Design review of the part built by this model. Coordinates are the model's own, in mm. Coordinates: 2 decimals unless noted, no trailing zeros. Loops run counter-clockwise (first coordinate to the right, second up) from the corner with the lowest first, then second, coordinate; pieces in that order, holes last. Notation, with made-up numbers: (71.5, 43) -> (101.5, 43) arc R27 cw to (101.5, 71) -> close; hole circle Ø2 at (30, -2.5). An arc over 180 degrees is marked (long way). Use a Markdown table: item, result. Add a question column.
Q1. For probe 1 along X at (y, z) = (-0.75, -127); probe 2 along Y at (x, z) = (278.5, -21.5); probe 3 along X at (y, z) = (-2, -63) (3 decimals), list the stretches that pass through material, from the lowest coordinate up.
Q2. Take a section at A-A on x = 1294. Write out the cut boundary in (y, z) (3 decimals), plus the area to 3 significant figures.
Q3. Clearance check with flat-ended pins moving along their axes: pin 1 Ø9 at (x, z) = (1057.275, -22.225) entering from -Y; pin 2 Ø2 at (y, z) = (-2, -117) entering from +X; pin 3 Ø1.3 at (x, y) = (677, 34) entering from -Z; pin 4 Ø8 at (x, z) = (930.275, -127) entering from +Y. State where each tip first meets the part, or that it passes through.
from build123d import *

# Parameters (mm, degrees)
BASE_FLANGE1_DEPTH               = 2.65684
EDGE_FLANGE3_STRIP_W             = 16.97736
EDGE_FLANGE3_STRIP_H             = 2.65684
EDGE_FLANGE3_STRIP_CUT_DEPTH     = 1409.7
EDGE_FLANGE3_DEPTH               = 1409.7
EDGE_FLANGE4_STRIP_W             = 16.97736
EDGE_FLANGE4_STRIP_H             = 2.65684
EDGE_FLANGE4_STRIP_CUT_DEPTH     = 1409.7
EDGE_FLANGE4_DEPTH               = 1409.7
F_10_0_1935_DIAMETER_HOLE1_D     = 4.9149
F_17_64_0_26563_DIAMETER_HOLE1_D = 6.747002
FILLET1_R                        = 3.175


# Sheet-metal steps are written as plain solids
with BuildPart() as part:
    # Sketch1 → Base-Flange1 (new body)
    with BuildSketch(Plane(origin=(0, 0, 0), x_dir=(1, 0, 0), z_dir=(0, 1, 0))):
        Polygon((0, 0), (1409.7, 0), (1409.7, 38.1), (996.95, 38.1), (958.85, 88.9), (958.85, 139.7), (920.75, 139.7), (920.75, 88.9), (882.65, 38.1), (527.05, 38.1), (488.95, 88.9), (488.95, 139.7), (450.85, 139.7), (450.85, 88.9), (412.75, 38.1), (0, 38.1), align=None)
    extrude(amount=-BASE_FLANGE1_DEPTH)

    # Edge-Flange3 strip (across the edge) → Edge-Flange3 strip cut (cut)
    with BuildSketch(Plane(origin=(0, 0, 0), x_dir=(0, 0, -1), z_dir=(1, 0, 0))):
        with Locations((-2.65684, -1.32842)):
            Rectangle(EDGE_FLANGE3_STRIP_W, EDGE_FLANGE3_STRIP_H)
    extrude(amount=EDGE_FLANGE3_STRIP_CUT_DEPTH, mode=Mode.SUBTRACT)

    # Edge-Flange3 section (across the edge) → Edge-Flange3 (add)
    with BuildSketch(Plane(origin=(0, 0, 0), x_dir=(0, 0, -1), z_dir=(1, 0, 0))):
        with BuildLine():
            Line((0, 3.175), (0, 35.44316))
            Line((0, 35.44316), (2.65684, 35.44316))
            Line((2.65684, 35.44316), (2.65684, 3.175))
            ThreePointArc((2.65684, 3.175), (3.58677597, 0.92993597), (5.83184, 0))
            Line((5.83184, 0), (5.83184, -2.65684))
            ThreePointArc((5.83184, -2.65684), (1.708106389, -0.948733611), (0, 3.175))
        make_face()
    extrude(amount=EDGE_FLANGE3_DEPTH)

    # Edge-Flange4 strip (across the edge) → Edge-Flange4 strip cut (cut)
    with BuildSketch(Plane(origin=(0, 35.44316, -2.65684), x_dir=(0, -1, 0), z_dir=(1, 0, 0))):
        with Locations((-2.65684, -1.32842)):
            Rectangle(EDGE_FLANGE4_STRIP_W, EDGE_FLANGE4_STRIP_H)
    extrude(amount=EDGE_FLANGE4_STRIP_CUT_DEPTH, mode=Mode.SUBTRACT)

    # Edge-Flange4 section (across the edge) → Edge-Flange4 (add)
    with BuildSketch(Plane(origin=(0, 35.44316, -2.65684), x_dir=(0, -1, 0), z_dir=(1, 0, 0))):
        with BuildLine():
            Line((0, 3.175), (0, 35.44316))
            Line((0, 35.44316), (2.65684, 35.44316))
            Line((2.65684, 35.44316), (2.65684, 3.175))
            ThreePointArc((2.65684, 3.175), (3.58677597, 0.92993597), (5.83184, 0))
            Line((5.83184, 0), (5.83184, -2.65684))
            ThreePointArc((5.83184, -2.65684), (1.708106389, -0.948733611), (0, 3.175))
        make_face()
    extrude(amount=EDGE_FLANGE4_DEPTH)

    # #10 (0.1935) Diameter Hole1 (through all)
    with Locations(Plane(origin=(0, -2.65684, 0), x_dir=(-1, 0, 0), z_dir=(0, -1, 0))):
        with Locations((-460.375, 127), (-479.425, 127), (-460.375, 63.5), (-479.425, 63.5), (-460.375, 95.25), (-479.425, 95.25), (-930.275, 63.5), (-949.325, 63.5), (-930.275, 95.25), (-949.325, 95.25), (-949.325, 127), (-930.275, 127)):
            Hole(F_10_0_1935_DIAMETER_HOLE1_D / 2)

    # 17/64 (0.26563) Diameter Hole1 (through all)
    with Locations(Plane(origin=(0, 35.44316, 0), x_dir=(1, 0, 0), z_dir=(0, 1, 0))):
        with Locations((22.225, 22.225), (1057.275, 22.225), (1387.475, 22.225), (352.425, 22.225)):
            Hole(F_17_64_0_26563_DIAMETER_HOLE1_D / 2)

    # Fillet1
    fillet1_edges = [part.edges().sort_by_distance(p)[0] for p in [
        (0, -1.32842, -38.1),
        (0, 34.11474, -38.1),
        (1409.7, 34.11474, -38.1),
        (1409.7, -1.32842, -38.1),
        (450.85, -1.32842, -139.7),
        (488.95, -1.32842, -139.7),
        (958.85, -1.32842, -139.7),
        (920.75, -1.32842, -139.7),
    ]]
    fillet(fillet1_edges, radius=FILLET1_R)


solid = part.part
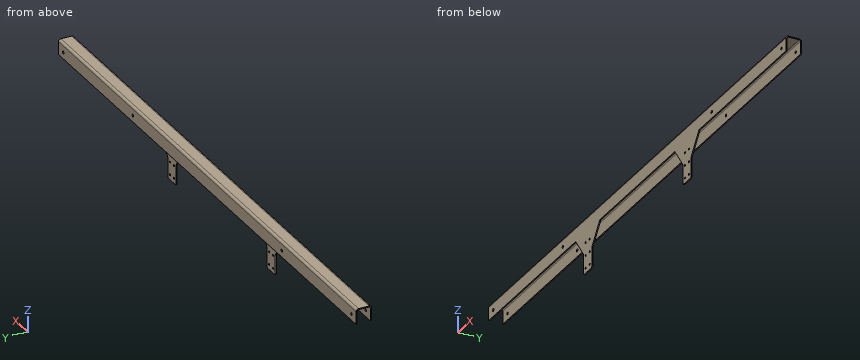
Answer list:
| question | item | result |
|---|---|---|
| 1 | probe 1 | 450.85 to 457.92, 462.83 to 476.97, 481.88 to 488.95, 920.75 to 927.82, 932.73 to 946.87, 951.78 to 958.85 |
| 1 | probe 2 | -2.66 to 0, 32.79 to 35.44 |
| 1 | probe 3 | 431.425 to 457.969, 462.781 to 477.019, 481.831 to 508.375, 901.325 to 927.869, 932.681 to 946.919, 951.731 to 978.275 |
| 2 | outline | (-2.657, -38.1) -> (0, -38.1) -> (0, -5.832) arc R3.175 cw to (3.175, -2.657) -> (29.611, -2.657) arc R3.175 cw to (32.786, -5.832) -> (32.786, -38.1) -> (35.443, -38.1) -> (35.443, -5.832) arc R5.832 ccw to (29.611, 0) -> (3.175, 0) arc R5.832 ccw to (-2.657, -5.832) -> close |
| 2 | area | 279 mm² |
| 3 | pin 1 | y = -2.66 |
| 3 | pin 2 | x = 958.85 |
| 3 | pin 3 | z = -38.1 |
| 3 | pin 4 | y = 0 |
